from build123d import *

# Parameters (mm, degrees)
F0_R            = 35.052
F0_R_2          = 19.0246
F1_DEPTH        = 53.848
F0_R_3          = 69.85
F0_R_4          = 53.848
F2_DEPTH        = 19.05
F3_R            = 3.048
F4_R            = 6.35
F5_DEPTH        = 19.051
F5_COPIES_COUNT = 4


# Not quite as in the source:
# - a pattern or mirror of a feature is missing from the dataset's text; its kind, count and spacing are read off the source's solid
# - a feature names something its author has since deleted; it is built from what else it names


with BuildPart() as f1:
    # F0 (on Front) → F1 (new body)
    with BuildSketch(Plane.XZ):
        Circle(F0_R)
        Circle(F0_R_2, mode=Mode.SUBTRACT)
    extrude(amount=F1_DEPTH)

    # F0 (on Front) → F2 (join)
    with BuildSketch(Plane.XZ):
        Circle(F0_R_3)
        Circle(F0_R_4, mode=Mode.SUBTRACT)
        Circle(F0_R_4)
        Circle(F0_R, mode=Mode.SUBTRACT)
    extrude(amount=F2_DEPTH)

    # F3
    f3_edges = [f1.edges().sort_by_distance(p)[0] for p in [
        (-69.85, -19.05, 0),
        (-69.85, 0, 0),
        (-35.052, -19.05, 0),
        (-35.052, -53.848, 0),
    ]]
    fillet(f3_edges, radius=F3_R)

    # F4 (on face) → F5 (cut, through all)
    with BuildSketch(Plane.XZ.offset(19.05)):
        with Locations((0, 53.848)):
            Circle(F4_R)
    f5 = extrude(amount=-F5_DEPTH, mode=Mode.SUBTRACT)

    # F5_copies: F5 ×4 about axis
    f5_copies_axis = Axis((0, 0, 0), (0, 1, 0))
    for i in range(1, F5_COPIES_COUNT):
        add(f5.rotate(f5_copies_axis, i * 360 / F5_COPIES_COUNT), mode=Mode.SUBTRACT)


solid = f1.part
CAD build for the part. Positions are in the model's coordinates, mm. A direction names the side the tool comes from. Give positions to 0.01 mm unless a question says otherwise; leave off trailing zeros. Order: outer loops, then holes, each group sorted by start corner. A loop starts at its lowest first (then second) coordinate and runs counter-clockwise, first axis right, second up. Notation, with made-up numbers: (13.5, 66.5) -> (18.5, 66.5) arc R15 cw to (18.5, 78.5) -> close; hole circle Ø8 at (39, 45). An arc over 180 degrees is marked (long way). Return JSON: item names as keys, results as strings.
Q1. Drill centre lines: line 1 (Z direction, x = 0, y = -6); line 2 (Z direction, x = -5, y = -15.5); line 3 (Y direction, x = -32.5, z = -40.5). Where is each one in solid material? Low to high.
Working result:
{"line 1": "-69.85 to -60.2, -47.5 to -19.02, 19.02 to 47.5, 60.2 to 69.85", "line 2": "-69.67 to -57.76, -49.93 to -18.36, 18.36 to 49.93, 57.76 to 69.67", "line 3": "-19.05 to 0"}
Q2. Flat gauge pins, fed straight in: pin 1 (8 mm diameter, centred on x = 6, z = 51, fed in from -Y); pin 2 (10 mm diameter, centred on x = 0, z = 53.848, fed in from +Y); pin 3 (10 mm diameter, centred on x = -35, z = 22, fed in from -Y); pin 4 (16.5 mm diameter, centred on x = 53.848, z = 0, fed in from +Y). Where does each tip first touch, or does it go through?
Working result:
{"pin 1": "y = -19.05", "pin 2": "through", "pin 3": "y = -19.61", "pin 4": "y = 0"}
Q3. Mould opens along X. For faces 3 (the face through (0.827, -9.658, -60.144)), 4 (the face through (33.433, -36.248, 10.529)), 5 (the face through (14, 0, -14)) say: pulls with the +X half, pulls with the -X half, needs draft (parallel to the pull), parting line crosses it, or undercut.
Working result:
{"face 3": "undercut", "face 4": "parting line crosses it", "face 5": "needs draft"}
Q4. Saw through at B-B (z = 0). Write the cut outline in (x, y), then the cut area to 3 significant figures.
Working result:
{"outline": "(-69.85, -16) arc R3.05 ccw to (-66.8, -19.05) -> (-60.2, -19.05) -> (-60.2, 0) -> (-66.8, 0) arc R3.05 ccw to (-69.85, -3.05) -> close; (-47.5, -19.05) -> (-38.1, -19.05) arc R3.05 cw to (-35.05, -22.1) -> (-35.05, -50.8) arc R3.05 ccw to (-32, -53.85) -> (-19.02, -53.85) -> (-19.02, 0) -> (-47.5, 0) -> close; (19.02, -53.85) -> (32, -53.85) arc R3.05 ccw to (35.05, -50.8) -> (35.05, -22.1) arc R3.05 cw to (38.1, -19.05) -> (47.5, -19.05) -> (47.5, 0) -> (19.02, 0) -> close; (60.2, -19.05) -> (66.8, -19.05) arc R3.05 ccw to (69.85, -16) -> (69.85, -3.05) arc R3.05 ccw to (66.8, 0) -> (60.2, 0) -> close", "area": "2,560 mm²"}
Q5. Which spindle directions (+Z, -Z, +X, -X, +Y, -Y) get a long thin tool onto all of the face, cutting with end or side? Do faces 1 (the face through (14, -53.848, -14)), 2 (the face through (29, -19.05, -29)). Say none if no direction does.
Working result:
{"face 1": "+Z, -Z, +X, -X, -Y", "face 2": "-Y"}
Q6. Saw through at D-D (y = -38). Write the cut outline in (x, z).
Working result:
{"outline": "circle Ø70.1 at (0, 0); hole circle Ø38.05 at (0, 0)"}
Q7. Saw through at A-A (x = 0). Write the cut outline in (y, z).
Working result:
{"outline": "(-53.85, -32) arc R3.05 ccw to (-50.8, -35.05) -> (-22.1, -35.05) arc R3.05 cw to (-19.05, -38.1) -> (-19.05, -47.5) -> (0, -47.5) -> (0, -19.02) -> (-53.85, -19.02) -> close; (-53.85, 19.02) -> (0, 19.02) -> (0, 47.5) -> (-19.05, 47.5) -> (-19.05, 38.1) arc R3.05 cw to (-22.1, 35.05) -> (-50.8, 35.05) arc R3.05 ccw to (-53.85, 32) -> close; (-19.05, -66.8) arc R3.05 ccw to (-16, -69.85) -> (-3.05, -69.85) arc R3.05 ccw to (0, -66.8) -> (0, -60.2) -> (-19.05, -60.2) -> close; (-19.05, 60.2) -> (0, 60.2) -> (0, 66.8) arc R3.05 ccw to (-3.05, 69.85) -> (-16, 69.85) arc R3.05 ccw to (-19.05, 66.8) -> close"}
Q8. Saw through at C-C (y = -11). Write the cut outline in (x, z).
Working result:
{"outline": "circle Ø139.7 at (0, 0); hole circle Ø12.7 at (-53.85, 0); hole circle Ø38.05 at (0, 0); hole circle Ø12.7 at (0, -53.85); hole circle Ø12.7 at (0, 53.85); hole circle Ø12.7 at (53.85, 0)"}
